from build123d import *

# Parameters (mm, degrees)
SKETCH_1_W          = 120
SKETCH_1_H          = 164
SKETCH_1_R          = 1.9
EXTRUDE_1_DEPTH     = 4
FILLET_1_R          = 15
SKETCH_2_W          = 110
SKETCH_2_H          = 5
EXTRUDE_2_DEPTH     = 30
CUT_EXTRUDE_1_REACH = 179.91
SKETCH_3_R          = 2.25
FILLET_2_R          = 5
FILLET_3_R          = 3
FILLET_4_R          = 3


# Some blends are built 0.0001 mm under size
with BuildPart() as part:
    # Эскиз1 → Бобышка-Вытянуть1 (new body)
    with BuildSketch(Plane(origin=(0, 0, 0), x_dir=(1, 0, 0), z_dir=(0, 1, 0))):
        Rectangle(SKETCH_1_W, SKETCH_1_H)
        with Locations(Location((-55, 55, 0), (0, 0, 270))):
            Circle(SKETCH_1_R, mode=Mode.SUBTRACT)
        with Locations(Location((55, 55, 0), (0, 0, 90))):
            Circle(SKETCH_1_R, mode=Mode.SUBTRACT)
        with Locations(Location((55, -55, 0), (0, 0, 270))):
            Circle(SKETCH_1_R, mode=Mode.SUBTRACT)
        with Locations(Location((-55, -55, 0), (0, 0, 90))):
            Circle(SKETCH_1_R, mode=Mode.SUBTRACT)
    extrude(amount=EXTRUDE_1_DEPTH)

    # Скругление1
    fillet_1_edges = [part.edges().sort_by_distance(p)[0] for p in [
        (60, 2, 82),
        (-60, 2, 82),
        (-60, 2, -82),
        (60, 2, -82),
    ]]
    fillet(fillet_1_edges, radius=FILLET_1_R)

    # Эскиз2 → Бобышка-Вытянуть2 (add)
    with BuildSketch(Plane(origin=(0, 4, 0), x_dir=(1, 0, 0), z_dir=(0, 1, 0))):
        with Locations((0, 79.5)):
            Rectangle(SKETCH_2_W, SKETCH_2_H)
        with Locations((0, -11.5)):
            Rectangle(SKETCH_2_W, SKETCH_2_H)
    extrude(amount=EXTRUDE_2_DEPTH)

    # Вырез-Вытянуть1: up to this face of the body (flat: up to its plane)
    cut_extrude_1_end = Plane(part.part.faces().sort_by_distance((0, 19, 14))[0])
    # Эскиз3 → Вырез-Вытянуть1 (cut, up to the picked face)
    with BuildSketch(Plane.XY.offset(-82), mode=Mode.PRIVATE) as cut_extrude_1_sk1:
        with Locations(Location((-45, 22, 0), (0, 0, 180))):
            Circle(SKETCH_3_R)
    cut_extrude_1_tool1 = split(extrude(cut_extrude_1_sk1.sketch, amount=CUT_EXTRUDE_1_REACH, mode=Mode.PRIVATE), bisect_by=cut_extrude_1_end, keep=Keep.BOTH, mode=Mode.PRIVATE)
    # Эскиз3 → Вырез-Вытянуть1 (cut, up to the picked face)
    with BuildSketch(Plane.XY.offset(-82), mode=Mode.PRIVATE) as cut_extrude_1_sk2:
        with Locations(Location((45, 22, 0), (0, 0, 180))):
            Circle(SKETCH_3_R)
    cut_extrude_1_tool2 = split(extrude(cut_extrude_1_sk2.sketch, amount=CUT_EXTRUDE_1_REACH, mode=Mode.PRIVATE), bisect_by=cut_extrude_1_end, keep=Keep.BOTH, mode=Mode.PRIVATE)
    add(cut_extrude_1_tool1.solids().sort_by(Axis((-45, 22, -82), (0, 0, 1)))[0], mode=Mode.SUBTRACT)
    add(cut_extrude_1_tool2.solids().sort_by(Axis((45, 22, -82), (0, 0, 1)))[0], mode=Mode.SUBTRACT)

    # Скругление2
    fillet_2_edges = [part.edges().sort_by_distance(p)[0] for p in [
        (55, 34, -79.5),
        (-55, 34, -79.5),
        (-55, 4, 11.5),
        (55, 4, 11.5),
        (-55, 34, 11.5),
        (55, 34, 11.5),
    ]]
    fillet(fillet_2_edges, radius=FILLET_2_R - 0.0001)  # a hair under: the kernel refuses the full size

    # Скругление3
    fillet_3_edges = [part.edges().sort_by_distance(p)[0] for p in [
        (0, 4, -77),
        (0, 4, 14),
        (0, 4, 9),
    ]]
    fillet(fillet_3_edges, radius=FILLET_3_R)

    # Скругление4
    # the kernel refuses this fillet: 3 mm, written as the material it adds along each edge
    with BuildSketch(Plane(origin=(-45, 4, -67), x_dir=(0.7513290268597076, 0, -0.659927794079053), z_dir=(0.659927794079053, 0, 0.7513290268597076))) as fillet_4_piece_1_section:
        with BuildLine():
            CenterArc((15 + FILLET_4_R, -FILLET_4_R), FILLET_4_R, 90, 90)
            Line((15, -FILLET_4_R), (15, 0))
            Line((15, 0), (15 + FILLET_4_R, 0))
        make_face()
    fillet_4_piece_1 = revolve(axis=Axis((-45, 4, -67), (0, 1, 0)), revolution_arc=119.166321534, mode=Mode.PRIVATE)
    fillet_4_piece_1 = split(fillet_4_piece_1, bisect_by=Plane(origin=(-45, 4, -82), z_dir=(0, 0, 1)), keep=Keep.TOP, mode=Mode.PRIVATE)
    fillet_4_piece_1 = split(fillet_4_piece_1, bisect_by=Plane(origin=(-55, 4, -67), z_dir=(1, 0, 0)), keep=Keep.TOP, mode=Mode.PRIVATE)
    add(fillet_4_piece_1)
    with BuildSketch(Plane(origin=(45, 4, -67), x_dir=(0.9424122347792039, 0, -0.33445355393307824), z_dir=(0.33445355393307824, 0, 0.9424122347792039))) as fillet_4_piece_2_section:
        with BuildLine():
            CenterArc((15 + FILLET_4_R, -FILLET_4_R), FILLET_4_R, 90, 90)
            Line((15, -FILLET_4_R), (15, 0))
            Line((15, 0), (15 + FILLET_4_R, 0))
        make_face()
    fillet_4_piece_2 = revolve(axis=Axis((45, 4, -67), (0, 1, 0)), revolution_arc=119.166321534, mode=Mode.PRIVATE)
    fillet_4_piece_2 = split(fillet_4_piece_2, bisect_by=Plane(origin=(45, 4, -82), z_dir=(0, 0, 1)), keep=Keep.TOP, mode=Mode.PRIVATE)
    fillet_4_piece_2 = split(fillet_4_piece_2, bisect_by=Plane(origin=(55, 4, -67), z_dir=(-1, 0, 0)), keep=Keep.TOP, mode=Mode.PRIVATE)
    add(fillet_4_piece_2)


solid = part.part
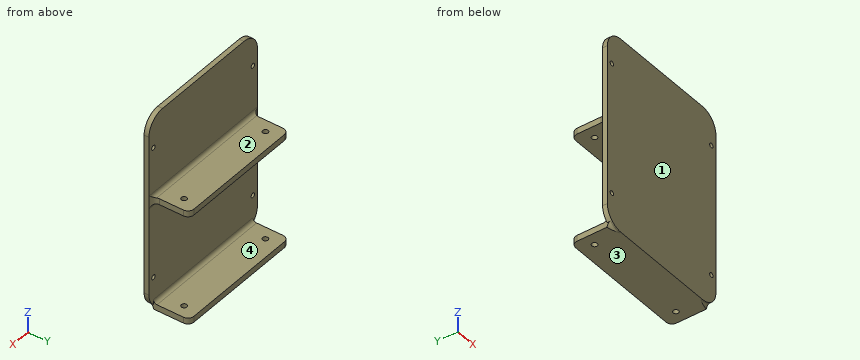
Model file for the job. Use its own axes, mm. Face numbers are marked on the shaded views. Round coordinates to 2 decimals unless told otherwise and drop trailing zeros. Order: outer loops, then holes, each group sorted by start corner. A loop starts at its lowest first (then second) coordinate and runs counter-clockwise, first axis right, second up.
(1) Band-saw the part on A-A (z = -55). List the corners of the cut face in (x, y).
(2) Band-saw the part on D-D (x = -33.5). List the corners of the cut face in (y, z), then the cut area to 3 significant figures.
(3) Pull direction Z, two halves, no side cores. Call the marked faces 1, 2, 3 and 4: released by +Z, released by -Z, zero draft, split by the parting line, or undercut.
(4) Band-saw the part on B-B (y = 22). List the corners of the cut face in (x, z), then the cut area to 3 significant figures.
(5) Band-saw the part on C-C (y = 13). List the corners of the cut face in (x, z).
(6) Pin check, flat tips, straight feed: pin 1 (3.5 mm diameter, centred on x = -45, y = 22, fed in from -Z); pin 2 (12 mm diameter, centred on x = -16, z = 28, fed in from +Y); pin 3 (7 mm diameter, centred on x = 45, y = 22, fed in from +Z); pin 4 (1.5 mm diameter, centred on y = 17.5, z = 11.5, fed in from -X). Stop position of each tip, or through.
(7) Drill centre lines: line 1 (X direction, y = 2, z = -55); line 2 (Z direction, x = 24.5, y = 27.5); line 3 (Y direction, x = 45, z = 11.9). Where is each one in solid material? Low to high.
Verdict:
1. outline: (-60, 0) - (-56.9, 0) - (-56.9, 4) - (-60, 4) - close; (-53.1, 0) - (53.1, 0) - (53.1, 4) - (-53.1, 4) - close; (56.9, 0) - (60, 0) - (60, 4) - (56.9, 4) - close
2. outline: (0, -82) - (34, -82) - (34, -77) - (7, -77) arc R3 cw to (4, -74) - (4, 6) arc R3 cw to (7, 9) - (34, 9) - (34, 14) - (7, 14) arc R3 cw to (4, 17) - (4, 82) - (0, 82) - close
2. area: 962 mm2
3. face 1: zero draft
3. face 2: released by +Z
3. face 3: released by -Z
3. face 4: undercut
4. outline: (-55, -82) - (-47.25, -82) - (-47.25, -77) - (-55, -77) - close; (-55, 9) - (-47.25, 9) - (-47.25, 14) - (-55, 14) - close; (-42.75, -82) - (42.75, -82) - (42.75, -77) - (-42.75, -77) - close; (-42.75, 9) - (42.75, 9) - (42.75, 14) - (-42.75, 14) - close; (47.25, -82) - (55, -82) - (55, -77) - (47.25, -77) - close; (47.25, 9) - (55, 9) - (55, 14) - (47.25, 14) - close
4. area: 1,010 mm2
5. outline: (-55, -82) - (55, -82) - (55, -77) - (-55, -77) - close; (-55, 9) - (55, 9) - (55, 14) - (-55, 14) - close
6. pin 1: passes through
6. pin 2: stops at y = 4
6. pin 3: stops at z = 14
6. pin 4: stops at x = -55
7. line 1: x = -60 to -56.9, -53.1 to 53.1, 56.9 to 60
7. line 2: z = -82 to -77, 9 to 14
7. line 3: y = 0 to 19.75, 24.25 to 34
